from build123d import *

# Parameters (mm, degrees)
CSK_FOR_M3_FLAT_HEAD_MACHINE_SCREW1_AT_2_COUNT = 2
CSK_FOR_M3_FLAT_HEAD_MACHINE_SCREW1_AT_2_PITCH = 13.856406460551039
CSK_FOR_M3_FLAT_HEAD_MACHINE_SCREW1_AT_3_COUNT = 2
CSK_FOR_M3_FLAT_HEAD_MACHINE_SCREW1_AT_3_PITCH = 13.856406460550982
ENL_V_MAT_EXTRU_1_DEPTH                        = 17.797023545854785
CONG_1_R                                       = 1


with BuildPart() as part:
    # Esquisse1 → Révolution1 (revolve)
    with BuildSketch(Plane.XY, mode=Mode.PRIVATE) as r_volution1_sk:
        Polygon((2.9999999999999996, -3.2), (2.9999999999999996, 3.2), (5.999999999999998, 3.2), (5.999999999999998, 2), (4.499999999999998, 2), (4.5, -1), (11.500000000000002, -1), (11.500000000000002, -3.2), align=None)
    revolve(r_volution1_sk.sketch.rotate(Axis((0, 4.689873417721518, 0), (0, -1, 0)), 90), axis=Axis((0, 4.689873417721518, 0), (0, -1, 0)))

    # Esquisse4 → CSK for M3 Flat Head Machine Screw1 (revolve, cut)
    with BuildSketch(Plane(origin=(-6.928203230275546, -1, 3.999999999999936), x_dir=(0, 0, 1), z_dir=(1, 0, 0))):
        Polygon((0, 0), (-5.4e-16, 2.2), (1.6999999999999995, 2.2), (1.6999999999999997, 1.3000000000000007), (3, 0), align=None)
    csk_for_m3_flat_head_machine_screw1 = revolve(axis=Axis((-6.928203230275546, 5.349999999999991, 3.999999999999936), (0, -1, 0)), mode=Mode.SUBTRACT)

    # CSK for M3 Flat Head Machine Screw1 at 2: CSK for M3 Flat Head Machine Screw1 ×2
    with Locations(*[(i * CSK_FOR_M3_FLAT_HEAD_MACHINE_SCREW1_AT_2_PITCH, 0, 0) for i in range(1, CSK_FOR_M3_FLAT_HEAD_MACHINE_SCREW1_AT_2_COUNT)]):
        add(csk_for_m3_flat_head_machine_screw1, mode=Mode.SUBTRACT)

    # CSK for M3 Flat Head Machine Screw1 at 3: CSK for M3 Flat Head Machine Screw1 ×2
    with Locations(*[Vector(0.5000000000000041, 0, -0.8660254037844364) * (i * CSK_FOR_M3_FLAT_HEAD_MACHINE_SCREW1_AT_3_PITCH) for i in range(1, CSK_FOR_M3_FLAT_HEAD_MACHINE_SCREW1_AT_3_COUNT)]):
        add(csk_for_m3_flat_head_machine_screw1, mode=Mode.SUBTRACT)

    # Esquisse6 → Enlèv. mat.-Extru.1 (cut, through all)
    with BuildSketch(Plane(origin=(0, -1, 0), x_dir=(1, 0, 0), z_dir=(0, 1, 0))):
        with BuildLine():
            Line((2.739426430539251, -3.5700900313105515), (3.348187859547974, -4.363443371601785))
            ThreePointArc((3.348187859547974, -4.363443371601785), (2.78e-15, -5.5), (-3.3481878595479704, -4.363443371601789))
            Line((-3.3481878595479704, -4.363443371601789), (-2.7394264305392486, -3.5700900313105546))
            ThreePointArc((-2.7394264305392486, -3.5700900313105546), (2.27e-15, -4.499999999999999), (2.739426430539251, -3.5700900313105515))
        make_face()
    extrude(amount=-ENL_V_MAT_EXTRU_1_DEPTH, mode=Mode.SUBTRACT)

    # Congé1
    # the kernel refuses this fillet: 1 mm, written as the material it takes off along each edge
    with BuildSketch(Plane(origin=(4.870091432069782, -3.2, 6.346826722329871), x_dir=(0.7933533402912335, 0, -0.608761429008723), z_dir=(-0.608761429008723, 0, -0.7933533402912334))) as cong_1_piece_1_section:
        with BuildLine():
            CenterArc((CONG_1_R, -CONG_1_R), CONG_1_R, 90, 90)
            Line((0, -CONG_1_R), (0, 0))
            Line((0, 0), (CONG_1_R, 0))
        make_face()
    cong_1_piece_1 = extrude(amount=6.0000000000000036, mode=Mode.PRIVATE)
    cong_1_piece_1 = cong_1_piece_1 - Plane(origin=(-8.9e-16, -2.973934992670689, -7.55e-15), x_dir=(-0.6087614290087209, 0, 0.7933533402912349), z_dir=(0, 1, 0)) * Cylinder(4.500000000000007, 17, mode=Mode.PRIVATE)
    cong_1_piece_1 = cong_1_piece_1 & Plane(origin=(-4.4e-16, -2.973934992670689, -1.78e-15), x_dir=(0.6087614290087225, 0, 0.7933533402912338), z_dir=(0, 1, 0)) * Cylinder(5.500000000000003, 17, mode=Mode.PRIVATE)
    add(cong_1_piece_1, mode=Mode.SUBTRACT)
    with BuildSketch(Plane(origin=(-1.2175228580174442, -3.2, 1.586706680582469), x_dir=(-0.7933533402912343, 0, -0.608761429008722), z_dir=(-0.6087614290087219, 0, 0.7933533402912343))) as cong_1_piece_2_section:
        with BuildLine():
            CenterArc((CONG_1_R, -CONG_1_R), CONG_1_R, 90, 90)
            Line((-9e-17, -CONG_1_R), (0, 0))
            Line((0, 0), (CONG_1_R, 0))
        make_face()
    cong_1_piece_2 = extrude(amount=6, mode=Mode.PRIVATE)
    cong_1_piece_2 = cong_1_piece_2 - Plane(origin=(-8.9e-16, -2.973934929539706, -7.55e-15), x_dir=(-0.6087614290087209, 0, 0.7933533402912349), z_dir=(0, 1, 0)) * Cylinder(4.500000000000007, 16, mode=Mode.PRIVATE)
    cong_1_piece_2 = cong_1_piece_2 & Plane(origin=(-4.4e-16, -2.973934929539706, -1.78e-15), x_dir=(0.6087614290087225, 0, 0.7933533402912338), z_dir=(0, 1, 0)) * Cylinder(5.500000000000003, 16, mode=Mode.PRIVATE)
    add(cong_1_piece_2, mode=Mode.SUBTRACT)
    with BuildSketch(Plane(origin=(-4.870091432069775, -1, 6.346826722329874), x_dir=(0, -1, 0), z_dir=(0.6087614290087219, 0, -0.7933533402912343))) as cong_1_piece_3_section:
        with BuildLine():
            CenterArc((CONG_1_R, CONG_1_R), CONG_1_R, 180.00000000000003, 90)
            Line((0, CONG_1_R), (0, 0))
            Line((0, 0), (CONG_1_R, 0))
        make_face()
    cong_1_piece_3 = extrude(amount=6, mode=Mode.PRIVATE)
    cong_1_piece_3 = cong_1_piece_3 - Plane(origin=(-8.9e-16, -1.2260647234530146, -7.55e-15), x_dir=(-0.6087614290087209, 0, 0.7933533402912349), z_dir=(0, 1, 0)) * Cylinder(4.500000000000007, 16, mode=Mode.PRIVATE)
    cong_1_piece_3 = cong_1_piece_3 & Plane(origin=(-4.4e-16, -1.2260647234530146, -1.78e-15), x_dir=(0.6087614290087225, 0, 0.7933533402912338), z_dir=(0, 1, 0)) * Cylinder(5.500000000000003, 16, mode=Mode.PRIVATE)
    add(cong_1_piece_3, mode=Mode.SUBTRACT)
    with BuildSketch(Plane(origin=(1.2175228580174433, -1, 1.586706680582468), x_dir=(2.1e-16, -1, -1.6e-16), z_dir=(0.608761429008723, 0, 0.7933533402912334))) as cong_1_piece_4_section:
        with BuildLine():
            CenterArc((CONG_1_R, CONG_1_R), CONG_1_R, 180, 90)
            Line((2.7e-16, CONG_1_R), (0, 0))
            Line((0, 0), (CONG_1_R, 0))
        make_face()
    cong_1_piece_4 = extrude(amount=6, mode=Mode.PRIVATE)
    cong_1_piece_4 = cong_1_piece_4 - Plane(origin=(-8.9e-16, -1.226064411710552, -7.55e-15), x_dir=(-0.6087614290087209, 0, 0.7933533402912349), z_dir=(0, 1, 0)) * Cylinder(4.500000000000007, 16, mode=Mode.PRIVATE)
    cong_1_piece_4 = cong_1_piece_4 & Plane(origin=(-4.4e-16, -1.226064411710552, -1.78e-15), x_dir=(0.6087614290087225, 0, 0.7933533402912338), z_dir=(0, 1, 0)) * Cylinder(5.500000000000003, 16, mode=Mode.PRIVATE)
    add(cong_1_piece_4, mode=Mode.SUBTRACT)


solid = part.part
Geometry: final body of the model. Coordinates: model frame, mm. A direction names the side the tool comes from. Coordinates: 2 decimals unless noted, no trailing zeros. Order: outer loops, then holes, each group sorted by start corner. A loop starts at its lowest first (then second) coordinate and runs counter-clockwise, first axis right, second up.
1) Section B-B (z = 0). Return loops of the section in (x, y), then the cut area to 3 significant figures.
Result sheet:
outline: (-11.5, -3.2) - (-3, -3.2) - (-3, 3.2) - (-6, 3.2) - (-6, 2) - (-4.5, 2) - (-4.5, -1) - (-11.5, -1) - close; (3, -3.2) - (11.5, -3.2) - (11.5, -1) - (4.5, -1) - (4.5, 2) - (6, 2) - (6, 3.2) - (3, 3.2) - close
area: 53.6 mm2
2) Set-up query: faces 1 (the flat face through (-4.5, 2, -1.4)), 2 (the cylindrical face through (3.25, -2.91, 3.75)), 3 (the cylindrical face through (5.49, -2.74, 4.91)), 4 (the flat face through (1, 3.2, 3)), 5 (the cylindrical face through (-1.802, 2.592, 5.723)). Return all of +Z, -Z, +X, -X, +Y, -Y with unobstructed straight access to the full face (end or side cutting, diameter ignored); none if empty.
Result sheet:
face 1: none
face 2: -Y
face 3: +Y, -Y
face 4: +Z, -Z, +X, -X, +Y
face 5: +Y
3) First-contact query: P1, Ø3, axis at x = 8, z = 8.5, coming from the +Y side; P2, Ø2, axis at x = -5.5, y = 1.5, coming from the -Z side; P3, Ø1, axis at y = -2.5, z = -6.5, coming from the -X side. Flat tips, straight axial feed; report the tip coordinate or a pass-through.
Result sheet:
P1: stops at y = -1
P2: stops at z = -3.81
P3: stops at x = -9.81
4) Section C-C (y = 0.5). Return loops of the section in (x, z).
Result sheet:
outline: circle Ø9 at (0, 0); hole circle Ø6 at (0, 0)
5) Ray query, probe 1 along X at (y, z) = (-2.75, 4); probe 2 along X at (y, z) = (-2.95, 4); probe 3 along X at (y, z) = (-1.25, 0). Return the intervals inside material, ascending.
Result sheet:
probe 1: x = -10.78 to -8.63, -5.23 to -3.28, -2.06 to 2.06, 3.28 to 5.23, 8.63 to 10.78
probe 2: x = -10.78 to -8.63, -5.23 to -3.5, -2.06 to 2.06, 3.5 to 5.23, 8.63 to 10.78
probe 3: x = -11.5 to -3, 3 to 11.5
6) Draft query along Y for faces 6 (the flat face through (2.4, -3.2, 2.4)), 7 (the cylindrical face through (-11.4, -2.1, -1.5)), 8 (the conical face through (2, -2, -8)), 9 (the cylindrical face through (3.2, -1.3, 3.7)). Return one class per face: released by +Y, released by -Y, zero draft, split by the parting line, or undercut.
Result sheet:
face 6: released by -Y
face 7: zero draft
face 8: undercut
face 9: undercut
7) Section A-A (x = 0). Return loops of the section in (y, z).
Result sheet:
outline: (-3.2, -11.5) - (-1, -11.5) - (-1, -11) - (-2.3, -9.7) - (-3.2, -9.7) - close; (-3.2, -6.3) - (-2.3, -6.3) - (-1, -5) - (-1, -4.5) - (2, -4.5) - (2, -6) - (3.2, -6) - (3.2, -3) - (-3.2, -3) - close; (-3.2, 3) - (3.2, 3) - (3.2, 6) - (2, 6) - (2, 4.5) - (-3.2, 4.5) - close; (-3.2, 5.5) - (-1, 5.5) - (-1, 11.5) - (-3.2, 11.5) - close
8) Section D-D (z = -4). Return loops of the section in (x, y), then the cut area to 3 significant figures.
Result sheet:
outline: (-10.78, -3.2) - (10.78, -3.2) - (10.78, -1) - (2.06, -1) - (2.06, 2) - (4.47, 2) - (4.47, 3.2) - (-4.47, 3.2) - (-4.47, 2) - (-2.06, 2) - (-2.06, -1) - (-10.78, -1) - close
area: 70.5 mm2
